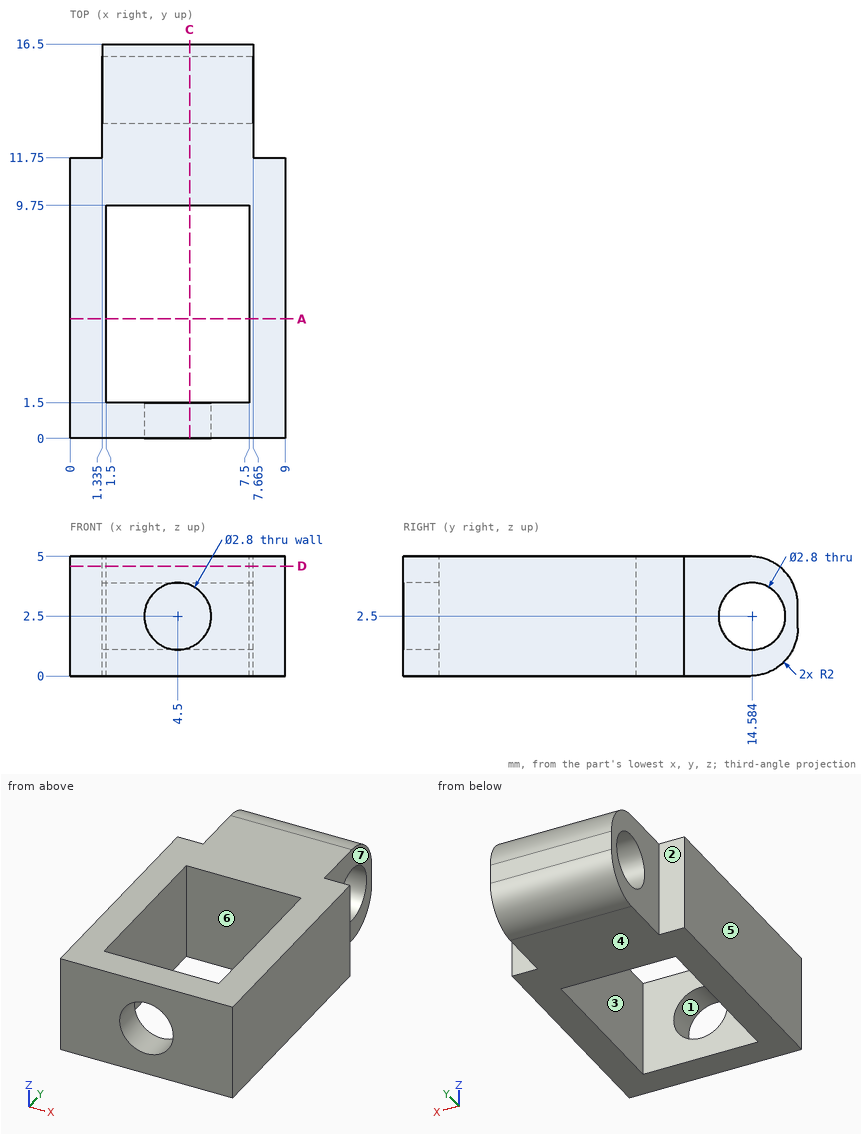
Source: three-view drawing plus pictorial views. Frame: mm from the lowest corner of the part. A direction names the side the tool comes from. Give positions to 0.01 mm unless a question says otherwise; leave off trailing zeros. Order: outer loops, then holes, each group sorted by start corner. A loop starts at its lowest first (then second) coordinate and runs counter-clockwise, first axis right, second up. Notation, with made-up numbers: M 10.5,26.25 L 53.5,26.25 A12 cw 53.5,33.25 Z; hole C 57,8.5 d3. An arc over 180 degrees is marked long. One line per question, with ' | ' between items. Start each with the question number.
1. First-contact query: pin 1 Ø1.4 at (y, z) = (13.5, 3.5) entering from +X (3 decimals); pin 2 Ø1.5 at (x, z) = (0.5, 2.5) entering from +Y; pin 3 Ø2.5 at (y, z) = (14.58, 2.5) entering from +X. Flat tips, straight axial feed; report the tip coordinate or a pass-through.
2. Material intervals for probe 1 along X at (y, z) = (5.75, 3.55); probe 2 along Y at (x, z) = (1.75, 1.6); probe 3 along Z at (x, y) = (4.5, 0.3), sorted ascending. Write a range as [from, to].
3. Access query for the marked faces 1, 2 and 3. Directions: +Z, -Z, +X, -X, +Y, -Y. A direction counts if a zero-diameter tool reaches every point of the face in a straight line with its end or side. Return the directions, or none.
4. Section query A-A (y = 5). Return the cut outline in (x, z).
5. Pull-direction query (X, two-part tool) for the marked faces 4, 5, 6 and 7; classes: released by +X, released by -X, zero draft, split by the parting line, or undercut.
6. Section query D-D (z = 4.6). Return the cut outline in (x, y) (3 decimals).
7. Section query C-C (x = 5). Return the cut outline in (y, z).
Here are the results:
1) pin 1: x = 7.665 | pin 2: y = 11.75 | pin 3: through
2) probe 1: [0, 1.5], [7.5, 9] | probe 2: [0, 1.5], [9.75, 13.51], [15.66, 16.46] | probe 3: [0, 1.1], [3.9, 5]
3) face 1: -Y | face 2: +Z, -Z, -X, +Y | face 3: +Z, -Z
4) outline: M 0,0 L 1.5,0 L 1.5,5 L 0,5 Z; M 7.5,0 L 9,0 L 9,5 L 7.5,5 Z
5) face 4: zero draft | face 5: released by -X | face 6: undercut | face 7: released by +X
6) outline: M 0,0 L 9,0 L 9,11.75 L 7.665,11.75 L 7.665,15.7 L 1.335,15.7 L 1.335,11.75 L 0,11.75 Z; hole M 1.5,1.5 L 7.5,1.5 L 7.5,9.75 L 1.5,9.75 Z
7) outline: M 0,0 L 1.5,0 L 1.5,1.19 L 0,1.19 Z; M 0,3.81 L 1.5,3.81 L 1.5,5 L 0,5 Z; M 9.75,0 L 14.5,0 A2 ccw 16.5,2 L 16.5,3 A2 ccw 14.5,5 L 9.75,5 Z; hole C 14.58,2.5 d2.8
